Can you work these out from the model? Positions are in its coordinate system, mm. Round coordinates to 2 decimals unless told otherwise and drop trailing zeros. Loops run counter-clockwise (first coordinate to the right, second up) from the corner with the lowest first, then second, coordinate; pieces in that order, holes last. Notation, with made-up numbers: (27, 10.5) -> (71, 10.5) arc R31 ccw to (71, 41.5) -> close; hole circle Ø11 at (-5.5, 63.5). An arc over 180 degrees is marked (long way). Write each question's results on one line, items separated by ' | '.
from build123d import *

# Parameters (mm, degrees)
SKETCH1_W           = 150
SKETCH1_H           = 48
BOSS_EXTRUDE1_DEPTH = 3
FILLET1_R           = 10
SKETCH2_R           = 0.8
CUT_EXTRUDE1_DEPTH  = 79.803553219
SKETCH3_R           = 1
CUT_EXTRUDE2_DEPTH  = 79.803553219


with BuildPart() as part:
    # Sketch1 → Boss-Extrude1 (new body)
    with BuildSketch(Plane(origin=(0, 0, 0), x_dir=(1, 0, 0), z_dir=(0, 1, 0))):
        Rectangle(SKETCH1_W, SKETCH1_H)
    extrude(amount=BOSS_EXTRUDE1_DEPTH)

    # Fillet1
    fillet1_edges = [part.edges().sort_by_distance(p)[0] for p in [
        (-75, 1.5, -24),
        (75, 1.5, -24),
        (75, 1.5, 24),
        (-75, 1.5, 24),
    ]]
    fillet(fillet1_edges, radius=FILLET1_R)

    # Sketch2 → Cut-Extrude1 (cut, through all)
    with BuildSketch(Plane(origin=(0, 3, 0), x_dir=(1, 0, 0), z_dir=(0, 1, 0))):
        with Locations(Location((-60, 0, 0), (0, 0, 270))):
            Circle(SKETCH2_R)
        with Locations(Location((60, 0, 0), (0, 0, 270))):
            Circle(SKETCH2_R)
    extrude(amount=-CUT_EXTRUDE1_DEPTH, mode=Mode.SUBTRACT)

    # Sketch3 → Cut-Extrude2 (cut, through all)
    with BuildSketch(Plane(origin=(0, 3, 0), x_dir=(1, 0, 0), z_dir=(0, 1, 0))):
        with Locations(Location((-8.5, 0, 0), (0, 0, 270))):
            Circle(SKETCH3_R)
        with Locations(Location((8.5, 0, 0), (0, 0, 270))):
            Circle(SKETCH3_R)
        with Locations(Location((0, 8.5, 0), (0, 0, 270))):
            Circle(SKETCH3_R)
        with Locations(Location((0, -8.5, 0), (0, 0, 270))):
            Circle(SKETCH3_R)
    extrude(amount=-CUT_EXTRUDE2_DEPTH, mode=Mode.SUBTRACT)


solid = part.part
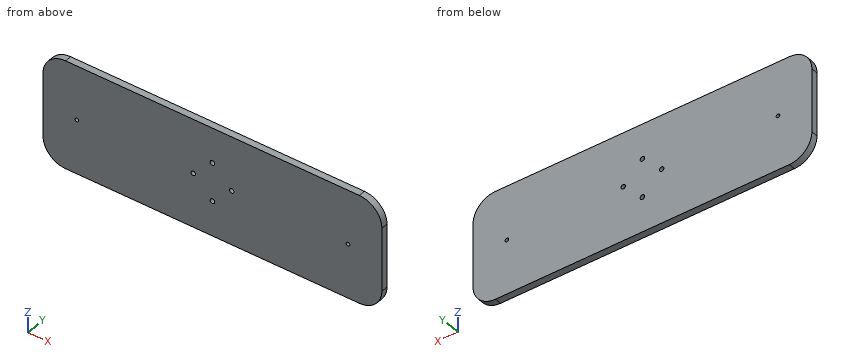
1. Will this pin go through, and if not, where does the flat tip stop? pin 1 (1.3 mm diameter, centred on x = 60, z = 0, fed in from +Y).
Final values:
pin 1: through
2. Please list where these lines run through material, in increasing order: line 1 (X direction, y = 0.85, z = 0); line 2 (Z direction, x = -60, y = 1.6); line 3 (X direction, y = 1.65, z = 8.5). Write a range as from..to.
Final values:
line 1: -75..-60.8, -59.2..-9.5, -7.5..7.5, 9.5..59.2, 60.8..75 | line 2: -24..-0.8, 0.8..24 | line 3: -75..-1, 1..75
3. If we section it at A-A (z = 20): List the corners of the cut face in (x, y) for me.
Final values:
outline: (-73, 0) -> (73, 0) -> (73, 3) -> (-73, 3) -> close
